```python
from build123d import *

# Parameters (mm, degrees)
F0_R          = 12
F1_DEPTH      = 5
F2_R          = 21
F3_DEPTH      = 12.001
F3_DEPTH_BACK = 12.001
F4_R          = 10.5
F5_DEPTH      = 6
F5_DEPTH_BACK = 4
F6_SIZE       = 2
F8_D          = 3
F8_DEPTH      = 8
F8_TIP        = 0.9012909285


with BuildPart() as f1:
    # F0 (on Right) → F1 (new body)
    with BuildSketch(Plane.YZ):
        Circle(F0_R)
    extrude(amount=F1_DEPTH)

    # F2 (on Top) → F3 (cut, two sides)
    with BuildSketch(Plane.XY) as f3_sk:
        with Locations((-17, 0)):
            Circle(F2_R)
    extrude(amount=-F3_DEPTH, mode=Mode.SUBTRACT)
    extrude(f3_sk.sketch, amount=F3_DEPTH_BACK, mode=Mode.SUBTRACT)

    # F4 (on Right) → F5 (join, two sides)
    with BuildSketch(Plane.YZ) as f5_sk:
        Circle(F4_R)
    extrude(amount=-F5_DEPTH)
    extrude(f5_sk.sketch, amount=F5_DEPTH_BACK)

    # F6
    f6_edges = [f1.edges().sort_by_distance(p)[0] for p in [
        (-6, -10.5, 0),
    ]]
    chamfer(f6_edges, length=F6_SIZE)

    # F8
    with Locations(Plane(origin=(-6, 0, 0), x_dir=(0, -1, 0), z_dir=(-1, 0, 0))):
        with Locations((0, 0)):
            Hole(F8_D / 2, depth=F8_DEPTH)
            with Locations((0, 0, -(F8_DEPTH + F8_TIP / 2))):  # 118° drill point
                Cone(0, F8_D / 2, F8_TIP, mode=Mode.SUBTRACT)


solid = f1.part
```
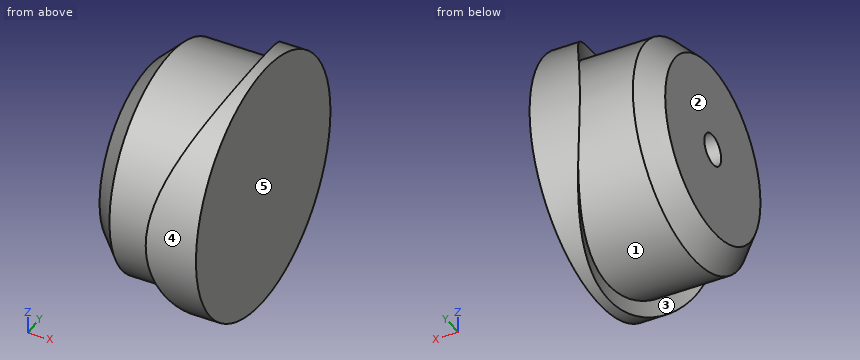
The listing builds one solid part. Answer for the finished solid, in the listing's coordinates (mm). Face numbers are marked on the shaded views. A direction names the side the tool comes from. Coordinates: 2 decimals unless noted, no trailing zeros. Write each loop counter-clockwise with the first axis right and the second up, starting at its lowest first coordinate (ties: lowest second). Pieces come first, ordered by that corner, then holes. Notation, with made-up numbers: (2.25, -35.75) - (34.25, -35.75) arc R18 ccw to (34.25, -1.75) - close; hole circle Ø4 at (-8, 17). An arc over 180 degrees is marked (long way). Return JSON: item names as keys, results as strings. Group by question number.
Q1. Find the intervals of material crossed by line 1 along Z through (x, y) = (0.25, 0); line 2 along Z through (x, y) = (-1.5, -0.75), in increasing order. Write a range as [from, to].
Q2. Which of the six approach directions +Z, -Z, +X, -X, +Y, -Y give full straight-line access (tool end or side, diameter ignored) to the marked faces 1 and 2?
Q3. The part is cut by section B-B on x = -3.25. Write down the section's boundary in (y, z), and give its area (3 significant figures).
Q4. For a pull along Y with two mould halves and no side action, classify the marked faces 3, 4 and 5 as +Y half, -Y half, draft (parallel to the pull), parting line (faces both ways), or undercut.
Q5. The part is cut by section A-A on x = -4.75. Write down the section's boundary in (y, z), and give its area (3 significant figures).
Q6. Flat-ended cylindrical pins translate along their axes: pin 1 Ø5 at (x, y) = (-5, 2) entering from +Z; pin 2 Ø1 at (y, z) = (7.5, 6) entering from -X; pin 3 Ø6 at (x, z) = (-1.5, -3.5) entering from -Y. Find the tip coordinate at first contact, or state that the pin passes through.
Evaluation:
{
 "1": {"line 1": "z = [-10.5, -1.5], [1.5, 10.5]", "line 2": "z = [-10.47, -1.3], [1.3, 10.47]"},
 "2": {"face 1": "-X", "face 2": "+Z, -Z, -X, +Y, -Y"},
 "3": {"outline": "circle Ø21 at (0, 0); hole circle Ø3 at (0, 0)", "area": "339 mm2"},
 "4": {"face 3": "undercut", "face 4": "parting line", "face 5": "draft"},
 "5": {"outline": "circle Ø19.5 at (0, 0); hole circle Ø3 at (0, 0)", "area": "292 mm2"},
 "6": {"pin 1": "stops at z = 10.5", "pin 2": "stops at x = -5.4", "pin 3": "stops at y = -11.95"}
}
